Geometry: final body of the model. Coordinates: model frame, mm. Round coordinates to 2 decimals unless told otherwise and drop trailing zeros. Loops run counter-clockwise (first coordinate to the right, second up) from the corner with the lowest first, then second, coordinate; pieces in that order, holes last. Notation, with made-up numbers: (30.5, 56.25) - (65.5, 56.25) arc R29 cw to (65.5, 83.25) - close; hole circle Ø11 at (-6, 64.5). An arc over 180 degrees is marked (long way). Use CSV: the item, a comma, the result in double quotes.
from build123d import *

# Parameters (mm, degrees)
SKETCH1_R                                       = 19.53
BOSS_EXTRUDE1_DEPTH                             = 1
CUT_EXTRUDE1_DEPTH                              = 28.637688036
CUT_EXTRUDE1_DEPTH_BACK                         = 28.637688036
SKETCH6_R                                       = 0.25
SKETCH6_R_2                                     = 1
CSK_FOR_M2_FLAT_HEAD_MACHINE_SCREW1_D           = 1
CSK_FOR_M2_FLAT_HEAD_MACHINE_SCREW1_CSINK_D     = 1.6
CSK_FOR_M2_FLAT_HEAD_MACHINE_SCREW1_CSINK_ANGLE = 100


with BuildPart() as part:
    # Sketch1 → Boss-Extrude1 (new body)
    with BuildSketch(Plane(origin=(0, 0, 0), x_dir=(1, 0, 0), z_dir=(0, 1, 0))):
        with Locations(Location((0, 0, 0), (0, 0, 270))):
            Circle(SKETCH1_R)
    extrude(amount=BOSS_EXTRUDE1_DEPTH)

    # Sketch6 → Cut-Extrude1 (cut, two sides: drawn at the far end of the back side and taken through both)
    with BuildSketch(Plane(origin=(0, 1, 0), x_dir=(1, 0, 0), z_dir=(0, 1, 0)).offset(-CUT_EXTRUDE1_DEPTH_BACK)):
        with Locations(Location((0, 10.25, 0), (0, 0, 270))):
            Circle(SKETCH6_R)
        with Locations(Location((7.778174593, 7.778174593, 0), (0, 0, 270))):
            Circle(SKETCH6_R_2)
    extrude(amount=CUT_EXTRUDE1_DEPTH + CUT_EXTRUDE1_DEPTH_BACK, mode=Mode.SUBTRACT)

    # CSK for M2 Flat Head Machine Screw1 (through all)
    with Locations(Plane(origin=(0, 1, 0), x_dir=(1, 0, 0), z_dir=(0, 1, 0))):
        with Locations((0, 14.29), (-14.29, 0), (0, -14.29), (14.29, 0)):
            CounterSinkHole(CSK_FOR_M2_FLAT_HEAD_MACHINE_SCREW1_D / 2, CSK_FOR_M2_FLAT_HEAD_MACHINE_SCREW1_CSINK_D / 2, counter_sink_angle=CSK_FOR_M2_FLAT_HEAD_MACHINE_SCREW1_CSINK_ANGLE)


solid = part.part
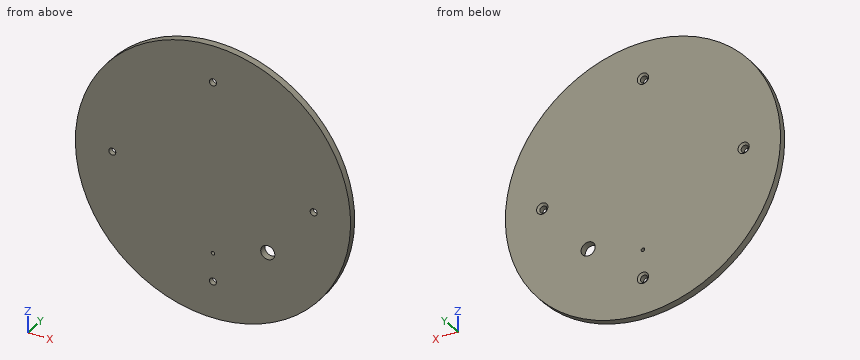
Item 1: Material intervals for line 1 (X direction, y = 0.7, z = -7.5); line 2 (X direction, y = 0.2, z = 14.29); line 3 (Z direction, x = -14, y = 0.2), sorted ascending.
Final values:
line 1,"x = -18.03 to 6.82, 8.74 to 18.03"
line 2,"x = -13.31 to -0.5, 0.5 to 13.31"
line 3,"z = -13.62 to -0.41, 0.41 to 13.62"
Item 2: Section D-D on x = -7.5. Return the cut outline in (y, z).
Final values:
outline,"(0, -18.03) - (1, -18.03) - (1, 18.03) - (0, 18.03) - close"
Item 3: Section A-A on x = 14.29. Return the cut outline in (y, z).
Final values:
outline,"(0, -13.31) - (1, -13.31) - (1, -0.8) - (0.75, -0.5) - (0, -0.5) - close; (0, 0.5) - (0.75, 0.5) - (1, 0.8) - (1, 13.31) - (0, 13.31) - close"
Item 4: Pin query (flat end, axial travel): P1, Ø1.6, axis at x = 7.78, z = -7.78, coming from the +Y side; P2, Ø2, axis at x = 1, z = -13, coming from the -Y side. Return the tip coordinate at first contact, or that it passes through.
Final values:
P1,"passes through"
P2,"stops at y = 0"
Item 5: Section B-B on z = 14.29. Return the cut outline in (x, y), plus the area to 3 significant figures.
Final values:
outline,"(-13.31, 0) - (-0.5, 0) - (-0.5, 0.75) - (-0.8, 1) - (-13.31, 1) - close; (0.5, 0) - (13.31, 0) - (13.31, 1) - (0.8, 1) - (0.5, 0.75) - close"
area,"25.5 mm²"
Item 6: Section C-C on y = 0.15. Return the cut outline in (x, z), plus the area to 3 significant figures.
Final values:
outline,"circle Ø39.06 at (0, 0); hole circle Ø1 at (-14.29, 0); hole circle Ø1 at (0, -14.29); hole circle Ø1 at (0, 14.29); hole circle Ø0.5 at (0, -10.25); hole circle Ø2 at (7.78, -7.78); hole circle Ø1 at (14.29, 0)"
area,"1,190 mm²"
